Build history of the part. All positions in model axes, mm. Face numbers are marked on the shaded views. Round coordinates to 2 decimals unless told otherwise and drop trailing zeros. Order: outer loops, then holes, each group sorted by start corner. A loop starts at its lowest first (then second) coordinate and runs counter-clockwise, first axis right, second up. Notation, with made-up numbers: (6, -8) -> (12, -8) arc R26 cw to (12, 13) -> close; hole circle Ø3 at (48, -25.75). An arc over 180 degrees is marked (long way). Answer as a JSON object with one key per item and string values.
from build123d import *

# Parameters (mm, degrees)
F0_R     = 62.5695627455
F1_DEPTH = 25.4
F2_T     = -2.54
F4_DEPTH = 5.08
F6_DEPTH = 5.08


with BuildPart() as f1:
    # F0 (on Front) → F1 (new body)
    with BuildSketch(Plane.XZ):
        Circle(F0_R)
    extrude(amount=F1_DEPTH)

    # F2
    f2_openings = [f1.faces().sort_by_distance(p)[0] for p in [
        (0, -25.4, 0),
    ]]
    offset(amount=F2_T, openings=f2_openings)

    # F3 (on face) → F4 (join)
    with BuildSketch(Plane.XZ.offset(2.54)):
        with BuildLine():
            Line((42.8714592834, 14.3697795653), (46.1623315652, 0.6234704811))
            Line((46.1623315652, 0.6234704811), (55.1577749403, 14.3697795653))
            Line((55.1577749403, 14.3697795653), (58.2842846629, 14.3697795653))
            ThreePointArc((58.2842846629, 14.3697795653), (-59.591645919, -7.2376888635), (60.0295627455, 0))
            ThreePointArc((60.0295627455, 0), (59.6196375987, 7.0033717604), (58.3954606874, 13.9110953747))
            Line((58.3954606874, 13.9110953747), (47.174907652, -2.5732086764))
            Line((47.174907652, -2.5732086764), (45.0967718461, -12.5282445057))
            Line((45.0967718461, -12.5282445057), (41.92952804, -12.5282445057))
            Line((41.92952804, -12.5282445057), (44.119518181, -2.4260319196))
            Line((44.119518181, -2.4260319196), (39.7454249692, 14.3697795653))
            Line((39.7454249692, 14.3697795653), (42.8714592834, 14.3697795653))
        make_face()
        with BuildLine():
            add(Edge.make_bspline(
                [(-35.7621383344, 10.6903606455), (-38.3053526918, 11.9560807539), (-40.8956636113, 11.9560807539)],
                knots=[0, 0, 0, 1, 1, 1], degree=2))
            add(Edge.make_bspline(
                [(-40.8956636113, 11.9560807539), (-44.098229839, 11.9560807539), (-46.6267265207, 10.1722984616)],
                knots=[0, 0, 0, 1, 1, 1], degree=2))
            add(Edge.make_bspline(
                [(-46.6267265207, 10.1722984616), (-49.1552232023, 8.3885161693), (-50.6358213756, 4.9386929902)],
                knots=[0, 0, 0, 1, 1, 1], degree=2))
            add(Edge.make_bspline(
                [(-50.6358213756, 4.9386929902), (-52.116419549, 1.488869811), (-52.116419549, -2.5732086764)],
                knots=[0, 0, 0, 1, 1, 1], degree=2))
            add(Edge.make_bspline(
                [(-52.116419549, -2.5732086764), (-52.116419549, -6.0171447853), (-50.3238066513, -8.0687887749)],
                knots=[0, 0, 0, 1, 1, 1], degree=2))
            add(Edge.make_bspline(
                [(-50.3238066513, -8.0687887749), (-48.5311937535, -10.1204327646), (-45.3874982285, -10.1204327646)],
                knots=[0, 0, 0, 1, 1, 1], degree=2))
            add(Edge.make_bspline(
                [(-45.3874982285, -10.1204327646), (-42.8266226604, -10.1204327646), (-39.459218465, -9.066647186)],
                knots=[0, 0, 0, 1, 1, 1], degree=2))
            Line((-39.459218465, -9.066647186), (-39.459218465, -11.8100219325))
            add(Edge.make_bspline(
                [(-39.459218465, -11.8100219325), (-41.0428403681, -12.3810677489), (-42.4792855143, -12.6400988408)],
                knots=[0, 0, 0, 1, 1, 1], degree=2))
            add(Edge.make_bspline(
                [(-42.4792855143, -12.6400988408), (-43.9157306606, -12.8991299328), (-45.9349957638, -12.8991299328)],
                knots=[0, 0, 0, 1, 1, 1], degree=2))
            add(Edge.make_bspline(
                [(-45.9349957638, -12.8991299328), (-50.3915079594, -12.8991299328), (-52.9288352464, -10.1469245808)],
                knots=[0, 0, 0, 1, 1, 1], degree=2))
            add(Edge.make_bspline(
                [(-52.9288352464, -10.1469245808), (-55.4661625335, -7.3947192288), (-55.4661625335, -2.6497405899)],
                knots=[0, 0, 0, 1, 1, 1], degree=2))
            add(Edge.make_bspline(
                [(-55.4661625335, -2.6497405899), (-55.4661625335, 2.1541087517), (-53.526372879, 6.2838885472)],
                knots=[0, 0, 0, 1, 1, 1], degree=2))
            add(Edge.make_bspline(
                [(-53.526372879, 6.2838885472), (-51.5865832245, 10.4136683428), (-48.3104286184, 12.5830537379)],
                knots=[0, 0, 0, 1, 1, 1], degree=2))
            add(Edge.make_bspline(
                [(-48.3104286184, 12.5830537379), (-45.0342740122, 14.7524391329), (-40.8956636113, 14.7524391329)],
                knots=[0, 0, 0, 1, 1, 1], degree=2))
            add(Edge.make_bspline(
                [(-40.8956636113, 14.7524391329), (-37.2751153942, 14.7524391329), (-34.496418226, 13.280671565)],
                knots=[0, 0, 0, 1, 1, 1], degree=2))
            Line((-34.496418226, 13.280671565), (-35.7621383344, 10.6903606455))
        make_face(mode=Mode.SUBTRACT)
        Polygon((-20.1790633255, -12.5282445057), (-21.2269618338, -3.974331401), (-30.3519207548, -3.974331401), (-34.8614165829, -12.5282445057), (-38.3406751134, -12.5282445057), (-23.6406606452, 14.3697795653), (-20.4380944174, 14.3697795653), (-17.0530290113, -12.5282445057), align=None, mode=Mode.SUBTRACT)
        with BuildLine():
            Line((11.3697462601, 14.3697795653), (5.6828363777, -12.5282445057))
            Line((5.6828363777, -12.5282445057), (2.3566416742, -12.5282445057))
            Line((2.3566416742, -12.5282445057), (-6.1089653764, 9.9721380724))
            Line((-6.1089653764, 9.9721380724), (-6.2149326412, 9.9721380724))
            add(Edge.make_bspline(
                [(-6.2149326412, 9.9721380724), (-6.8036396684, 5.9041725147), (-7.5807329443, 2.2836242977)],
                knots=[0, 0, 0, 1, 1, 1], degree=2))
            Line((-7.5807329443, 2.2836242977), (-10.7420896801, -12.5282445057))
            Line((-10.7420896801, -12.5282445057), (-13.7209472375, -12.5282445057))
            Line((-13.7209472375, -12.5282445057), (-8.0399244254, 14.3697795653))
            Line((-8.0399244254, 14.3697795653), (-4.7255038625, 14.3697795653))
            Line((-4.7255038625, 14.3697795653), (3.716554907, -8.0776193803))
            Line((3.716554907, -8.0776193803), (3.8284092421, -8.0776193803))
            add(Edge.make_bspline(
                [(3.8284092421, -8.0776193803), (4.3817938477, -3.9566701902), (5.1530000532, -0.6245884165)],
                knots=[0, 0, 0, 1, 1, 1], degree=2))
            Line((5.1530000532, -0.6245884165), (8.355566281, 14.3697795653))
            Line((8.355566281, 14.3697795653), (11.3697462601, 14.3697795653))
        make_face(mode=Mode.SUBTRACT)
        with BuildLine():
            add(Edge.make_bspline(
                [(32.4660625784, 11.6175742133), (35.1064135952, 8.8653688613), (35.1064135952, 3.6082151088)],
                knots=[0, 0, 0, 1, 1, 1], degree=2))
            add(Edge.make_bspline(
                [(35.1064135952, 3.6082151088), (35.1064135952, -1.1956342328), (33.1725110109, -4.8750531526)],
                knots=[0, 0, 0, 1, 1, 1], degree=2))
            add(Edge.make_bspline(
                [(33.1725110109, -4.8750531526), (31.2386084267, -8.5544720723), (27.6533826313, -10.541358289)],
                knots=[0, 0, 0, 1, 1, 1], degree=2))
            add(Edge.make_bspline(
                [(27.6533826313, -10.541358289), (24.0681568359, -12.5282445057), (19.2466462835, -12.5282445057)],
                knots=[0, 0, 0, 1, 1, 1], degree=2))
            Line((19.2466462835, -12.5282445057), (12.7708689847, -12.5282445057))
            Line((12.7708689847, -12.5282445057), (18.4518917968, 14.3697795653))
            Line((18.4518917968, 14.3697795653), (24.7451699171, 14.3697795653))
            add(Edge.make_bspline(
                [(24.7451699171, 14.3697795653), (29.8257115615, 14.3697795653), (32.4660625784, 11.6175742133)],
                knots=[0, 0, 0, 1, 1, 1], degree=2))
        make_face(mode=Mode.SUBTRACT)
    extrude(amount=F4_DEPTH)

    # F5 (on face) → F6 (join)
    with BuildSketch(Plane.XZ.offset(2.54)):
        Polygon((-22.1393704414, 7.7067422681), (-27.1837823093, 0), (-22.1393704414, 0), align=None)
    extrude(amount=F6_DEPTH)


solid = f1.part
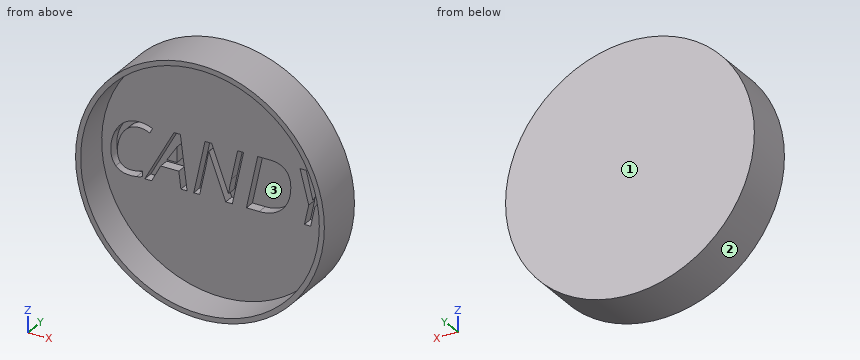
1) Probe L1, parallel to Z at x = 0, y = -16.25; L2, parallel to Y at x = 2, z = -38; L3, parallel to X at y = -12.25, z = 37. List the from-to ranges inside material, lowest first. Write a range as from..to.
Checked values:
{"L1": "z = -62.57..-60.03, 60.03..62.57", "L2": "y = -7.62..0", "L3": "x = -50.46..-47.27, 47.27..50.46"}
2) Cut at A-A, the plane y = -4.75. Count the separate pieces of the cut face and the enclosed holes in it, plus the area to 3 significant figures.
Checked values:
{"separate pieces": "2", "enclosed holes": "5", "area": "11,100 mm²"}
3) Flat gauge pins, fed straight in: pin 1 Ø2.5 at (y, z) = (-6, 2.5) entering from +X; pin 2 Ø1.5 at (x, y) = (9.5, -6) entering from -Z; pin 3 Ø6 at (x, y) = (23, -5) entering from +Z. Where does each tip first touch, or does it go through?
Checked values:
{"pin 1": "stops at x = 62.56", "pin 2": "stops at z = -61.95", "pin 3": "stops at z = 59.29"}
4) Cut at D-D, the plane z = 23. Give the cut face in (x, y).
Checked values:
{"outline": "(-58.19, -25.4) -> (-55.45, -25.4) -> (-55.45, -7.62) -> (55.45, -7.62) -> (55.45, -25.4) -> (58.19, -25.4) -> (58.19, 0) -> (-58.19, 0) -> close"}
5) Pull direction Z, two halves, no side cores. Call the marked faces 1, 2 and 3: pulls with the +Z half, pulls with the -Z half, needs draft (parallel to the pull), parting line crosses it, or undercut.
Checked values:
{"face 1": "needs draft", "face 2": "parting line crosses it", "face 3": "undercut"}
6) Cut at B-B, the plane y = -16.5. Give the cut face in (x, z), plus the area to 3 significant figures.
Checked values:
{"outline": "circle Ø125.14 at (0, 0); hole circle Ø120.06 at (0, 0)", "area": "978 mm²"}
7) Cut at C-C, the plane x = 0. Give the cut face in (y, z), plus the area to 3 significant figures.
Checked values:
{"outline": "(-25.4, -62.57) -> (0, -62.57) -> (0, 62.57) -> (-25.4, 62.57) -> (-25.4, 60.03) -> (-7.62, 60.03) -> (-7.62, 1.8) -> (-2.54, 1.8) -> (-2.54, -6.26) -> (-7.62, -6.26) -> (-7.62, -60.03) -> (-25.4, -60.03) -> close", "area": "1,000 mm²"}
